Verification items for this drawing (mm, ordinates from the low corner). A direction names the side the tool comes from. Round coordinates to 2 decimals unless told otherwise and drop trailing zeros. Loops run counter-clockwise (first coordinate to the right, second up) from the corner with the lowest first, then second, coordinate; pieces in that order, holes last. Notation, with made-up numbers: M 33.5,-21.5 L 91.5,-21.5 A11 cw 91.5,-3.5 Z; hole C 88.5,30.5 d4. An arc over 180 degrees is marked long. Write item = value, one per line.
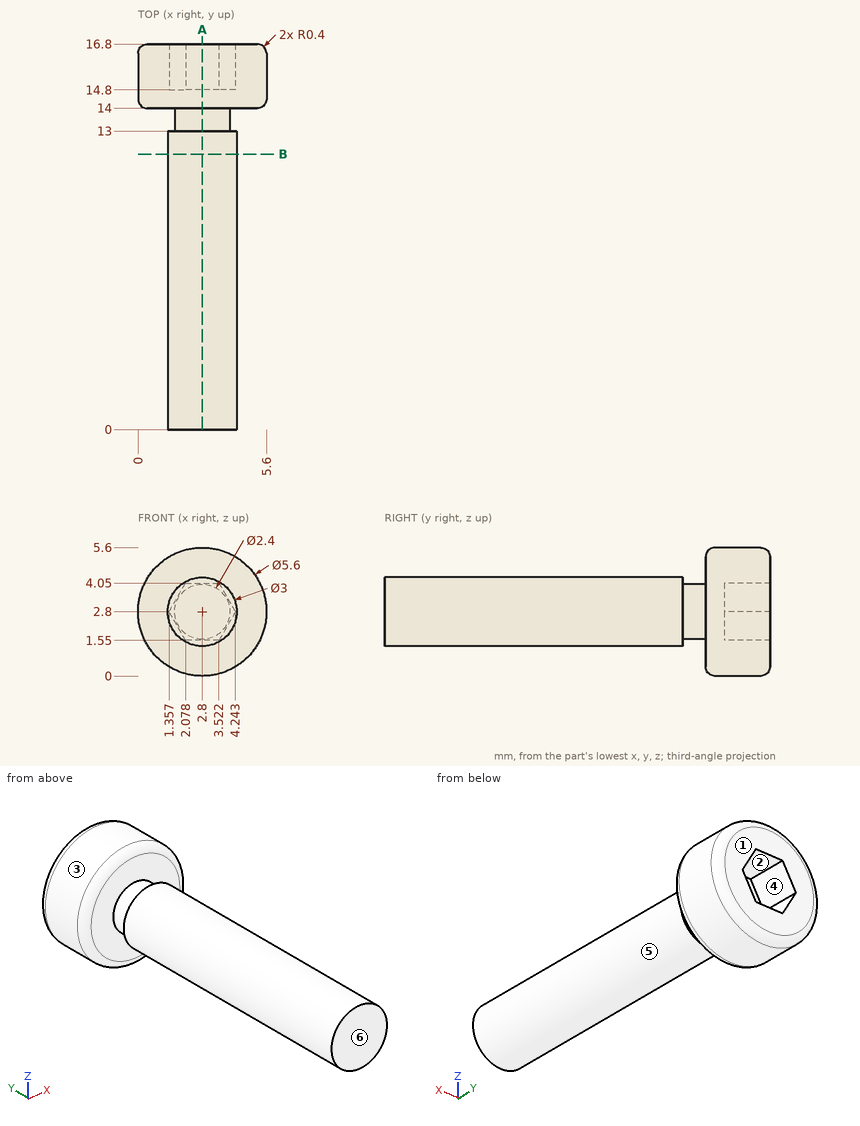
(1) Material ranges on line 1 along Y through (x, z) = (1.25, 3.55); line 2 along Y through (x, z) = (3.4, 3.6); line 3 along Z through (x, y) = (2.75, 3), recorded low to high. Write a range as from..to.
Result set:
line_1 = 14..16.8
line_2 = 0..14.8
line_3 = 1.3..4.3
(2) Depth check by flat-ended pin: pin 1 Ø1.5 at (x, y) = (3.5, 13.5) entering from +Z; pin 2 Ø2 at (x, y) = (4.5, 7) entering from -Z; pin 3 Ø0.8 at (x, z) = (3.5, 3) entering from +Y. Enter the tip coordinate at first touch or a pass-through.
Result set:
pin_1 = 5.51
pin_2 = 1.47
pin_3 = 14.8
(3) Release check for a two-part mould opening along Z. For the marked faces 1, 2 and 3 record: released by +Z, released by -Z, zero draft, split by the parting line, or undercut.
Result set:
face_1 = zero draft
face_2 = undercut
face_3 = split by the parting line
(4) Sectioned sample at B-B on y = 12. Record the cut outline in (x, z).
Result set:
outline = C 2.8,2.8 d3
(5) Tool access check on the marked faces 4, 5 and 6. Record the directions out of +Z, -Z, +X, -X, +Y, -Y that give a thin tool (end or side, any length) a straight path to the whole face; none if there is none.
Result set:
face_4 = +Y
face_5 = -Y
face_6 = +Z, -Z, +X, -X, -Y
(6) Sectioned sample at A-A on x = 2.8. Record the cut outline in (y, z).
Result set:
outline = M 0,1.3 L 13,1.3 L 13,1.6 L 14,1.6 L 14,0.4 A0.4 ccw 14.4,0 L 16.4,0 A0.4 ccw 16.8,0.4 L 16.8,1.55 L 14.8,1.55 L 14.8,4.05 L 16.8,4.05 L 16.8,5.2 A0.4 ccw 16.4,5.6 L 14.4,5.6 A0.4 ccw 14,5.2 L 14,4 L 13,4 L 13,4.3 L 0,4.3 Z
